The figure shows three views and two pictorial views of one solid part (mm, origin at its lowest corner). Answer the questions. Coordinates: 2 decimals unless noted, no trailing zeros. Order: outer loops, then holes, each group sorted by start corner. A loop starts at its lowest first (then second) coordinate and runs counter-clockwise, first axis right, second up. Notation, with made-up numbers: (69, 63) - (115, 63) arc R34 ccw to (115, 99) - close; hole circle Ø11 at (0.25, 22.25). An arc over 180 degrees is marked (long way). Use one line per item in the form item = value. Start each with the question number.
Item 1: Section B-B, the plane z = 102 is taken. Write down the section's boundary in (x, y), and give its area (3 significant figures).
Item 2: Consider line 1 along X through (y, z) = (112.5, 265); line 2 along Y through (x, z) = (372.5, 12); line 3 along Z through (x, y) = (339, 9.5). Determine where each line is inside the solid, lowest interval first. Write a range as [from, to].
Item 3: This flat-tipped pin is pushed along its axis until it touches: pin 1 Ø7.5 at (y, z) = (122.5, 159.5) entering from -X. Where does it stop, or does it pass through?
Item 4: Section A-A, the plane y = 100 is taken. Write down the section's boundary in (x, z), and give its area (3 significant figures).
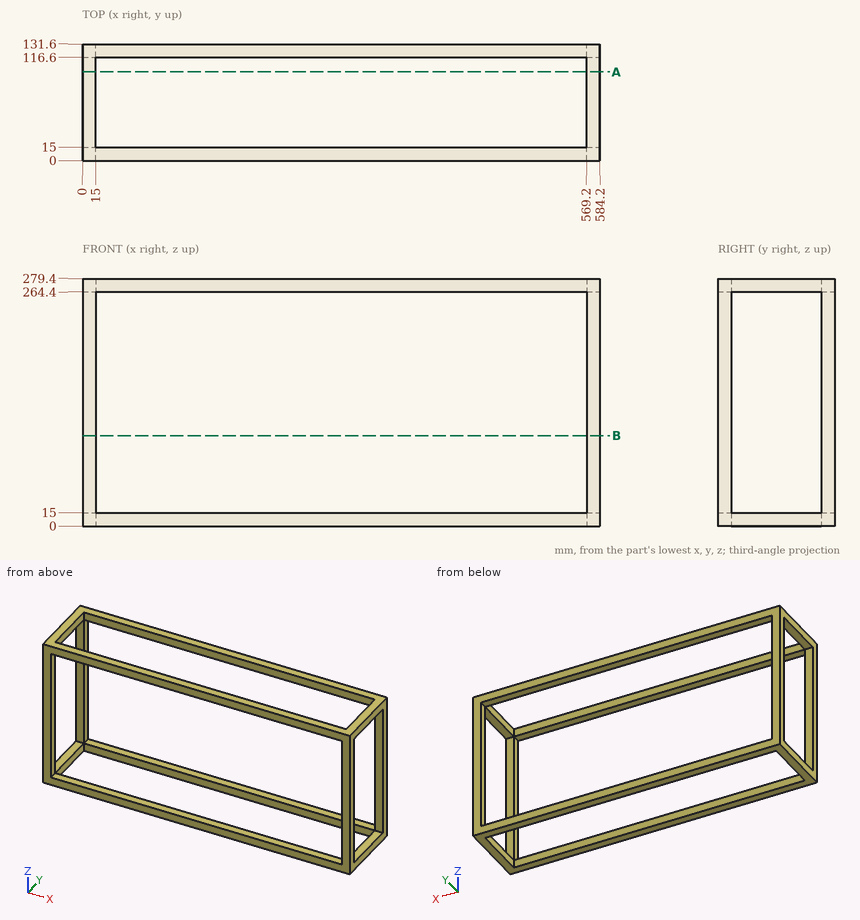
Response:
q1.outline = (0, 0) - (15, 0) - (15, 15) - (0, 15) - close; (0, 116.6) - (15, 116.6) - (15, 131.6) - (0, 131.6) - close; (569.2, 0) - (584.2, 0) - (584.2, 15) - (569.2, 15) - close; (569.2, 116.6) - (584.2, 116.6) - (584.2, 131.6) - (569.2, 131.6) - close
q1.area = 900 mm2
q2.line_1 = [0, 15], [569.2, 584.2]
q2.line_2 = [0, 15], [116.6, 131.6]
q2.line_3 = [0, 15], [264.4, 279.4]
q3.pin_1 = 0
q4.outline = (0, 0) - (15, 0) - (15, 15) - (0, 15) - close; (0, 264.4) - (15, 264.4) - (15, 279.4) - (0, 279.4) - close; (569.2, 0) - (584.2, 0) - (584.2, 15) - (569.2, 15) - close; (569.2, 264.4) - (584.2, 264.4) - (584.2, 279.4) - (569.2, 279.4) - close
q4.area = 900 mm2
